Here's how the part is built. I have some questions about the finished solid (model axes, mm). A direction names the side the tool comes from. Give positions to 0.01 mm unless a question says otherwise; leave off trailing zeros. Loops run counter-clockwise (first coordinate to the right, second up) from the corner with the lowest first, then second, coordinate; pieces in that order, holes last. Notation, with made-up numbers: (13.25, 75) -> (40.25, 75) arc R31 cw to (40.25, 103) -> close; hole circle Ø6 at (80, -10.75). An arc over 180 degrees is marked (long way). Answer in a Markdown table with one row per item. Add a question column.
Item 1: For P1, Ø3, axis at y = 20, z = 2, coming from the -X side; P2, Ø14.5, axis at x = -3, y = -2, coming from the +Z side, each with a flat end and sliding along its axis, tell me the tip position at first contact or that it passes through.
Item 2: If we section it at A-A (y = -19): Write out the boundary of the cut face in (x, z), then the cut area to 4 significant figures.
Item 3: If we section it at C-C (x = 4.5): Write out the boundary of the cut face in (y, z), then the cut area to 3 significant figures.
Item 4: If we section it at B-B (z = 3.25): Write out the boundary of the cut face in (x, y).
Item 5: We'd pull the mould along Y, two halves only. Please class faces 1 (the face through (18.174, 25.952, 2.465)), 2 (the face through (-1, -28.022, 3)), 3 (the face through (24.845, -5, 2)): released by +Y, released by -Y, zero draft, split by the parting line, or undercut.
Item 6: If I drill on line 1 (Y direction, x = -7, z = 2.7); line 2 (X direction, y = -5, z = 3.8); line 3 (Z direction, x = -1, y = 15), over which ranges is the centre line in solid material (lowest first)?
Item 7: Which directions (+Z, -Z, +X, -X, +Y, -Y) give clear straight access to the entire face, cutting with the end or side of a thin tool? Please do faces 4 (the face through (-1, 1, 1)), 5 (the face through (24, -1, 5)).
Item 8: If we section it at D-D (x = 10.5): Write out the boundary of the cut face in (y, z), then the cut area to 3 significant figures.
```python
from build123d import *

# Parameters (mm, degrees)
PAD026_DEPTH    = 5
POCKET005_DEPTH = 4
SKETCH030_W     = 19.322021
SKETCH030_H     = 8.266103
POCKET006_DEPTH = 5


with BuildPart() as part:
    # Sketch028 → Pad026 (new body)
    with BuildSketch(Plane.XY):
        Polygon((-13.074139, 32.516678), (-26.638874, 19.106085), (-26.638874, -29.449505), (24.845465, -29.449505), (24.845465, 19.568523), (11.313561, 32.516678), align=None)
    extrude(amount=PAD026_DEPTH)

    # Sketch029 (on Face8 of Pad026) → Pocket005 (cut)
    with BuildSketch(Plane.XY.offset(5)):
        Polygon((-25.033306, 18.464409), (-13.081248, 29.420872), (11.783705, 29.420872), (23.004097, 17.85417), (23.004097, -28.02212), (-25.033306, -28.02212), align=None)
    extrude(amount=-POCKET005_DEPTH, mode=Mode.SUBTRACT)

    # Sketch030 (on Face4 of Pocket005) → Pocket006 (cut)
    with BuildSketch(Plane(origin=(0, 0, 0), x_dir=(1, 0, 0), z_dir=(0, 0, -1))):
        with Locations((-0.2128295, 18.4669375)):
            Rectangle(SKETCH030_W, SKETCH030_H)
    extrude(amount=-POCKET006_DEPTH, mode=Mode.SUBTRACT)


solid = part.part
```
Recorded:
| question | item | result |
|---|---|---|
| 1 | P1 | stops at x = -26.64 |
| 1 | P2 | stops at z = 1 |
| 2 | outline | (-26.64, 0) -> (-9.87, 0) -> (-9.87, 1) -> (-25.03, 1) -> (-25.03, 5) -> (-26.64, 5) -> close; (9.45, 0) -> (24.85, 0) -> (24.85, 5) -> (23, 5) -> (23, 1) -> (9.45, 1) -> close |
| 2 | area | 45.95 mm^2 |
| 3 | outline | (-29.45, 0) -> (-22.6, 0) -> (-22.6, 1) -> (-28.02, 1) -> (-28.02, 5) -> (-29.45, 5) -> close; (-14.33, 0) -> (32.52, 0) -> (32.52, 5) -> (29.42, 5) -> (29.42, 1) -> (-14.33, 1) -> close |
| 3 | area | 71.8 mm^2 |
| 4 | outline | (-26.64, -29.45) -> (24.85, -29.45) -> (24.85, 19.57) -> (11.31, 32.52) -> (-13.07, 32.52) -> (-26.64, 19.11) -> close; hole (-25.03, -28.02) -> (23, -28.02) -> (23, 17.85) -> (11.78, 29.42) -> (-13.08, 29.42) -> (-25.03, 18.46) -> close |
| 5 | face 1 | released by +Y |
| 5 | face 2 | undercut |
| 5 | face 3 | zero draft |
| 6 | line 1 | y = -29.45 to -28.02, 29.42 to 32.52 |
| 6 | line 2 | x = -26.64 to -25.03, 23 to 24.85 |
| 6 | line 3 | z = 0 to 1 |
| 7 | face 4 | +Z |
| 7 | face 5 | +Z, +X, -X, +Y, -Y |
| 8 | outline | (-29.45, 0) -> (32.52, 0) -> (32.52, 5) -> (29.42, 5) -> (29.42, 1) -> (-28.02, 1) -> (-28.02, 5) -> (-29.45, 5) -> close |
| 8 | area | 80.1 mm^2 |
